from build123d import *

# Parameters (mm, degrees)
F0_W      = 150
F0_H      = 140
F1_DEPTH  = 2
F3_DEPTH  = 2.001
F5_DEPTH  = 2.001
F7_DEPTH  = 2.001
F8_R      = 50
F9_DEPTH  = 1
F11_DEPTH = 25


with BuildPart() as f1:
    # F0 (on Top) → F1 (new body)
    with BuildSketch(Plane.XY):
        Rectangle(F0_W, F0_H)
    extrude(amount=F1_DEPTH)

    # F2 (on face) → F3 (cut, through all)
    with BuildSketch(Plane.XY.offset(2)):
        Polygon((-75, 70), (-75, 41.5), (-46.5, 70), align=None)
        Polygon((-46.5, -70), (-75, -41.5), (-75, -70), align=None)
    extrude(amount=-F3_DEPTH, mode=Mode.SUBTRACT)

    # F4 (on face) → F5 (cut, through all)
    with BuildSketch(Plane.XY.offset(2)):
        with BuildLine():
            Line((-69.68, 9.5), (-75, 9.5))
            Line((-75, 9.5), (-75, -9.5))
            Line((-75, -9.5), (-69.68, -9.5))
            ThreePointArc((-69.68, -9.5), (-67.912233047, -8.767766953), (-67.18, -7))
            Line((-67.18, -7), (-67.18, 7))
            ThreePointArc((-67.18, 7), (-67.912233047, 8.767766953), (-69.68, 9.5))
        make_face()
    extrude(amount=-F5_DEPTH, mode=Mode.SUBTRACT)

    # F6 (on face) → F7 (cut, through all)
    with BuildSketch(Plane.XY.offset(2)):
        with BuildLine():
            Line((-28.0316714603, -70), (-15, -70))
            Line((-15, -70), (-16.4167693452, -66.4955507391))
            ThreePointArc((-16.4167693452, -66.4955507391), (-21.5158357302, -63.056987617), (-26.6149021151, -66.4955507391))
            Line((-26.6149021151, -66.4955507391), (-28.0316714603, -70))
        make_face()
        with BuildLine():
            Line((-27.8761372256, 70), (-26.6312305576, 66.430881427))
            ThreePointArc((-26.6312305576, 66.430881427), (-21.4380686128, 62.742253563), (-16.244906668, 66.430881427))
            Line((-16.244906668, 66.430881427), (-15, 70))
            Line((-15, 70), (-27.8761372256, 70))
        make_face()
    extrude(amount=-F7_DEPTH, mode=Mode.SUBTRACT)

    # F8 (on face) → F9 (join)
    with BuildSketch(Plane.XY.offset(2)):
        with Locations((-3.16, 0)):
            Circle(F8_R)
    extrude(amount=F9_DEPTH)

    # F10 (on face) → F11 (cut)
    with BuildSketch(Plane.XY.offset(3)):
        with BuildLine():
            Line((-3.6879379587, 7.8371274476), (-3.6960266549, 49.9971266717))
            ThreePointArc((-3.6960266549, 49.9971266717), (-36.7261918512, 37.05820779), (-52.8603788952, 5.4655592283))
            Line((-52.8603788952, 5.4655592283), (-10.9972216764, 0.4713958675))
            Line((-10.9972216764, 0.4713958675), (-10.9972216764, -0.5286041325))
            Line((-10.9972216764, -0.5286041325), (-53.1572216493, -0.5270933046))
            ThreePointArc((-53.1572216493, -0.5270933046), (-40.550995441, -33.1950818636), (-9.6065138215, -49.5826830612))
            Line((-9.6065138215, -49.5826830612), (-4.6131023208, -7.7194361544))
            Line((-4.6131023208, -7.7194361544), (-3.6201410564, -7.8378757061))
            Line((-3.6201410564, -7.8378757061), (-3.6208964704, -49.9978756993))
            ThreePointArc((-3.6208964704, -49.9978756993), (30.0356406829, -37.3904993234), (46.5405422428, -5.4640736429))
            Line((46.5405422428, -5.4640736429), (4.6772058717, -0.4714122399))
            Line((4.6772058717, -0.4714122399), (4.6772058717, 0.5285877601))
            Line((4.6772058717, 0.5285877601), (46.8372058717, 0.5285877601))
            ThreePointArc((46.8372058717, 0.5285877601), (33.9001692932, 33.5640261584), (2.3039733451, 49.7005532694))
            Line((2.3039733451, 49.7005532694), (-2.6879379587, 7.8371274476))
            Line((-2.6879379587, 7.8371274476), (-3.6879379587, 7.8371274476))
        make_face()
    extrude(amount=-F11_DEPTH, mode=Mode.SUBTRACT)


solid = f1.part
Input: part model. Units: mm. Frame: model coordinates. A direction names the side the tool comes from. Coordinates: 2 decimals unless noted, no trailing zeros. Write each loop counter-clockwise with the first axis right and the second up, starting at its lowest first coordinate (ties: lowest second). Pieces come first, ordered by that corner, then holes. Notation, with made-up numbers: M 64.25,47 L 79.25,47 A19 cw 79.25,79 Z; hole C 48.5,23.5 d1. An arc over 180 degrees is marked long. Answer as a JSON object with one key per item and string values. Group by question number.
(1) Ray query, line 1 along X through (y, z) = (43, 1.6); line 2 along X through (y, z) = (21.5, 0.2); line 3 along Y through (x, z) = (-3, 1.5). Return the intervals inside material, ascending. Write a range as [from, to].
(2) Section A-A on z = 2.55. Output: boundary loops of the cut face in (x, y).
(3) Contact query for flat-ended pins moving along their axis: P1, Ø1, axis at y = 1.5, z = 1.5, coming from the -X side; P2, Ø1, axis at x = -71.5, z = 1, coming from the +Y side; P3, Ø1.6, axis at x = -72.5, z = 1.5, coming from the -Y side. Output: stop coordinate, or through.
(4) Section C-C on x = -38. Output: boundary loops of the cut face in (y, z), plus the area to 3 significant figures.
(5) Section B-B on y = -35. Output: boundary loops of the cut face in (x, z), plus the area to 3 significant figures.
(6) Set-up query: faces 1 (the face through (49, 1, 2)), 2 (the face through (-21.533, 62.743, 1.014)), 3 (the face through (25.902, -3.003, 1.521)). Return all of +Z, -Z, +X, -X, +Y, -Y with unobstructed straight access to the full face (end or side cutting, diameter ignored); none if empty.
(7) Section D-D on x = 57. Output: boundary loops of the cut face in (y, z), plus the area to 3 significant figures.
Result set:
{
 "1": {"line 1": "x = [-73.5, -28.67], [-3.69, 1.5], [22.35, 75]", "line 2": "x = [-75, -48.3], [-3.69, -1.06], [41.98, 75]", "line 3": "y = [-70, -50], [7.84, 70]"},
 "2": {"outline": "M -53.16,-0.53 L -11,-0.53 L -11,0.47 L -52.86,5.47 A50 ccw Z; M -9.61,-49.58 A50 ccw -3.62,-50 L -3.62,-7.84 L -4.61,-7.72 Z; M -3.7,50 L -3.69,7.84 L -2.69,7.84 L 2.3,49.7 A50 ccw Z; M 4.68,-0.47 L 46.54,-5.46 A50 ccw 46.84,0.53 L 4.68,0.53 Z"},
 "3": {"P1": "stops at x = -67.18", "P2": "stops at y = 45.5", "P3": "stops at y = -44.8"},
 "4": {"outline": "M -70,0 L -35.86,0 L -35.86,2 L -70,2 Z; M -0.53,0 L 3.69,0 L 3.69,3 L -0.53,3 Z; M 35.86,0 L 70,0 L 70,2 L 35.86,2 Z", "area": "149 mm2"},
 "5": {"outline": "M -75,0 L -38.87,0 L -38.87,2 L -75,2 Z; M -7.87,0 L -3.62,0 L -3.62,3 L -7.87,3 Z; M 32.55,0 L 75,0 L 75,2 L 32.55,2 Z", "area": "170 mm2"},
 "6": {"face 1": "+Z", "face 2": "+Z, -Z, +Y", "face 3": "+Z, -Z"},
 "7": {"outline": "M -70,0 L 70,0 L 70,2 L -70,2 Z", "area": "280 mm2"}
}
